Geometry: final body of the model. Coordinates: model frame, mm. A direction names the side the tool comes from. Round coordinates to 2 decimals unless told otherwise and drop trailing zeros. Order: outer loops, then holes, each group sorted by start corner. A loop starts at its lowest first (then second) coordinate and runs counter-clockwise, first axis right, second up. Notation, with made-up numbers: (6, 50.25) -> (14, 50.25) arc R16 ccw to (14, 63.25) -> close; hole circle Ø9 at (69, 8.5). An arc over 180 degrees is marked (long way). Put each result on its own line as item: value.
```python
from build123d import *

# Parameters (mm, degrees)
F1_DEPTH    = 1.9558
F2_SIZE2    = 2.8438227154
F2_SIZE     = 0.762
F2_2_SIZE2  = 2.8438227154
F2_2_SIZE   = 0.762
F3_R        = 0.1950302499
F4_T1_DEPTH = 4.1020358569
F4_T4_ANGLE = 90
F4_T6_ANGLE = 90


# Not quite as in the source:
# - a fillet or chamfer that OpenCascade refuses, or shapes differently, is made with other operations: its cross-section is extruded or revolved along the edge and cut away or added


with BuildPart() as f1:
    # F0 (on Front) → F1 (new body)
    with BuildSketch(Plane.XZ):
        Polygon((-37.9921731242, 36.4987568722), (-48.2858929149, 36.4987568722), (-48.2858929149, 34.1091437473), (-48.2858929149, 29.5576006174), (-47.5840330195, 29.5576006174), (-47.5840330195, 34.1091437473), (-43.1390330195, 34.1091437473), (-38.6940330195, 34.1091437473), (-38.6940330195, 29.5576006174), (-37.9921731242, 29.5576006174), (-37.9921731242, 34.1091437473), align=None)
    extrude(amount=F1_DEPTH)

    # F2
    f2_edges = [f1.edges().sort_by_distance(p)[0] for p in [
        (-47.934963, -1.9558, 29.557601),
    ]]
    f2_side = f1.faces().sort_by_distance((-47.934963, -0.9779, 29.557601))[0]
    chamfer(f2_edges, length=F2_SIZE, length2=F2_SIZE2, reference=f2_side)

    # F2#2
    f2_2_edges = [f1.edges().sort_by_distance(p)[0] for p in [
        (-38.343103, -1.9558, 29.557601),
    ]]
    f2_2_side = f1.faces().sort_by_distance((-38.343103, -0.9779, 29.557601))[0]
    chamfer(f2_2_edges, length=F2_2_SIZE, length2=F2_2_SIZE2, reference=f2_2_side)

    # F3
    f3_edges = [f1.edges().sort_by_distance(p)[0] for p in [
        (-47.934963, -1.1938, 29.557601),
        (-38.343103, -1.1938, 29.557601),
        (-37.992173, -1.5748, 30.979512),
        (-38.694033, -1.5748, 30.979512),
        (-38.343103, -1.9558, 32.401423),
        (-43.139033, -1.9558, 34.109144),
        (-47.584033, -1.5748, 30.979512),
        (-48.285893, -1.5748, 30.979512),
        (-47.934963, -1.9558, 32.401423),
        (-47.584033, -1.9558, 33.255284),
        (-38.694033, -1.9558, 33.255284),
        (-37.992173, -1.9558, 34.45009),
        (-38.694033, -0.5969, 29.557601),
        (-37.992173, -0.5969, 29.557601),
        (-38.694033, -0.9779, 34.109144),
        (-47.584033, -0.9779, 34.109144),
        (-47.584033, -0.5969, 29.557601),
        (-48.285893, -0.5969, 29.557601),
        (-48.285893, -1.9558, 34.45009),
        (-43.139033, -1.9558, 36.498757),
    ]]
    fillet(f3_edges, radius=F3_R)

    # F4: fillet of radius 0.8584943428 on 2 edges, made by hand

    # F4_s2 → F4_t1 (cut)
    with BuildSketch(Plane.XZ.offset(-2.1462358569)):
        with BuildLine():
            ThreePointArc((-37.9921731242, 35.6402625294), (-38.2436202956, 36.2473097008), (-38.850667467, 36.4987568722))
            Line((-38.850667467, 36.4987568722), (-37.9921731242, 36.4987568722))
            Line((-37.9921731242, 36.4987568722), (-37.9921731242, 35.6402625294))
        make_face()
        with BuildLine():
            ThreePointArc((-47.4273985721, 36.4987568722), (-48.0344457435, 36.2473097008), (-48.2858929149, 35.6402625294))
            Line((-48.2858929149, 35.6402625294), (-48.2858929149, 36.4987568722))
            Line((-48.2858929149, 36.4987568722), (-47.4273985721, 36.4987568722))
        make_face()
    extrude(amount=F4_T1_DEPTH, mode=Mode.SUBTRACT)

    # F4_s3 → F4_t4 (revolve, cut)
    with BuildSketch(Plane.YZ.offset(-47.4273985721)):
        with BuildLine():
            ThreePointArc((-1.9558, 36.3037266223), (-1.8986769623, 36.4416338345), (-1.7607697501, 36.4987568722))
            Line((-1.7607697501, 36.4987568722), (-1.9558, 36.4987568722))
            Line((-1.9558, 36.4987568722), (-1.9558, 36.3037266223))
        make_face()
    revolve(axis=Axis((-47.4273985721, -1.9558, 35.6402625294), (0, -1, 0)), revolution_arc=F4_T4_ANGLE, mode=Mode.SUBTRACT)

    # F4_s5 → F4_t6 (revolve, cut)
    with BuildSketch(Plane.XY.offset(35.6402625294)):
        with BuildLine():
            ThreePointArc((-38.1872033741, -1.9558), (-38.0492961619, -1.8986769623), (-37.9921731242, -1.7607697501))
            Line((-37.9921731242, -1.7607697501), (-37.9921731242, -1.9558))
            Line((-37.9921731242, -1.9558), (-38.1872033741, -1.9558))
        make_face()
    revolve(axis=Axis((-38.850667467, -1.9558, 35.6402625294), (0, -1, 0)), revolution_arc=F4_T6_ANGLE, mode=Mode.SUBTRACT)


solid = f1.part
```
1. Cut plane A-A on z = 33.75. Return loops of the section in (x, y), and give its area (3 significant figures).
Ans:
outline: (-48.29, -1.76) arc R0.2 ccw to (-48.09, -1.96) -> (-47.78, -1.96) arc R0.2 ccw to (-47.58, -1.76) -> (-47.58, 0) -> (-48.29, 0) -> close; (-38.69, -1.76) arc R0.2 ccw to (-38.5, -1.96) -> (-38.19, -1.96) arc R0.2 ccw to (-37.99, -1.76) -> (-37.99, 0) -> (-38.69, 0) -> close
area: 2.71 mm²
2. Material intervals for probe 1 along X at (y, z) = (-1.65, 33.75); probe 2 along Z at (x, y) = (-45.75, -0.8); probe 3 along Y at (x, z) = (-40, 34.25), sorted ascending.
Ans:
probe 1: -48.29 to -47.58, -38.69 to -37.99
probe 2: 34.11 to 36.5
probe 3: -1.95 to 0
3. Draft query along X for faces 3 (the face through (-48.03, -0.87, 36.25)), 4 (the face through (-43, -1, 34.109)), 5 (the face through (-43, 0, 35)). Return one class per face: +X half, -X half, draft (parallel to the pull), parting line (faces both ways), or undercut.
Ans:
face 3: -X half
face 4: undercut
face 5: draft
4. Set-up query: faces 1 (the face through (-38.2, -0.9, 36.2)), 2 (the face through (-38.694, -1, 32)). Return all of +Z, -Z, +X, -X, +Y, -Y with unobstructed straight access to the full face (end or side cutting, diameter ignored); none if empty.
Ans:
face 1: +Z, +X, +Y, -Y
face 2: -Z, +Y, -Y
5. Cut plane C-C on x = -43.75. Return loops of the section in (y, z), and give its area (3 significant figures).
Ans:
outline: (-1.96, 34.3) arc R0.2 ccw to (-1.76, 34.11) -> (0, 34.11) -> (0, 36.5) -> (-1.76, 36.5) arc R0.2 ccw to (-1.96, 36.3) -> close
area: 4.66 mm²
6. Cut plane B-B on y = -0.7. Return loops of the section in (x, z), and give its area (3 significant figures).
Ans:
outline: (-48.29, 29.75) arc R0.2 ccw to (-48.09, 29.56) -> (-47.78, 29.56) arc R0.2 ccw to (-47.58, 29.75) -> (-47.58, 33.91) arc R0.2 cw to (-47.39, 34.11) -> (-38.89, 34.11) arc R0.2 cw to (-38.69, 33.91) -> (-38.69, 29.75) arc R0.2 ccw to (-38.5, 29.56) -> (-38.19, 29.56) arc R0.2 ccw to (-37.99, 29.75) -> (-37.99, 35.64) arc R0.86 ccw to (-38.85, 36.5) -> (-47.43, 36.5) arc R0.86 ccw to (-48.29, 35.64) -> close
area: 30.7 mm²
7. Contact query for flat-ended pins moving along their axis: P1, Ø0.9, axis at x = -43.5, y = -1, coming from the -Z side; P2, Ø1, axis at x = -42.5, z = 32, coming from the +Y side. Output: stop coordinate, or through.
Ans:
P1: z = 34.11
P2: through
